Here's the drawing with two shaded views (mm, measured from the low corner). I have some questions. A direction names the side the tool comes from. Coordinates: 2 decimals unless noted, no trailing zeros. Write each loop counter-clockwise with the first axis right and the second up, starting at its lowest first coordinate (ties: lowest second). Pieces come first, ordered by that corner, then holes. Notation, with made-up numbers: (80, 19.5) -> (93, 19.5) arc R23 cw to (93, 36.5) -> close; hole circle Ø1 at (1, 51.25). An arc over 180 degrees is marked (long way). Use one line per item in the form item = value.
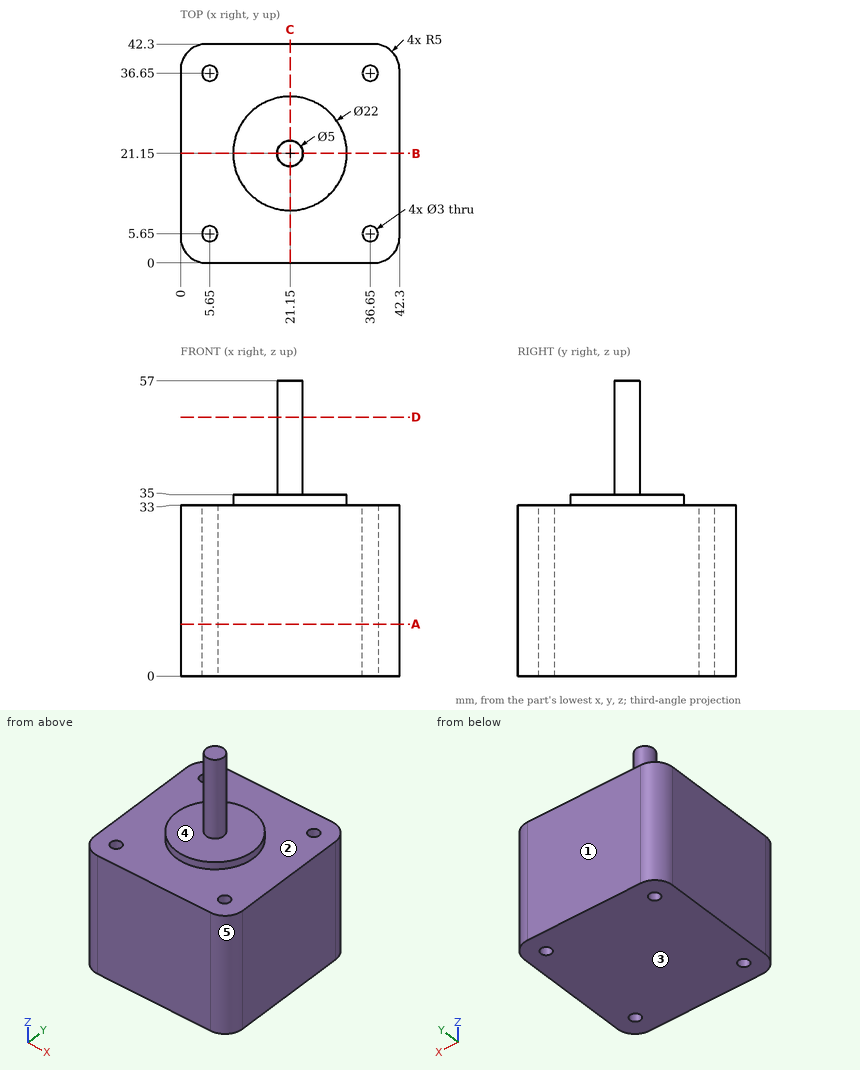
Q1. Thinking about a two-plate mould opening in Z: for the marked faces 3, 4 and 5, which applies, released by +Z, released by -Z, zero draft, split by the parting line, or undercut?
Return value:
face_3 = released by -Z
face_4 = released by +Z
face_5 = zero draft
Q2. For the marked faces 1 and 2, which set-ups out of +Z, -Z, +X, -X, +Y, -Y let a thin tool reach every point of the face, with its end or its side?
Return value:
face_1 = +Z, -Z, +X, -X, +Y
face_2 = +Z
Q3. Suppose I cut it at B-B (y = 21.15). Write out the boundary of the cut face in (x, z), then the cut area to 3 significant figures.
Return value:
outline = (0, 0) -> (42.3, 0) -> (42.3, 33) -> (32.15, 33) -> (32.15, 35) -> (23.65, 35) -> (23.65, 57) -> (18.65, 57) -> (18.65, 35) -> (10.15, 35) -> (10.15, 33) -> (0, 33) -> close
area = 1,550 mm2
Q4. Suppose I cut it at D-D (z = 50). Write out the boundary of the cut face in (x, y).
Return value:
outline = circle Ø5 at (21.15, 21.15)
Q5. Will these pins go through, and if not, where does the flat tip stop? pin 1 (10 mm diameter, centred on x = 18, z = 41.5, fed in from -Y); pin 2 (12 mm diameter, centred on x = 10, z = 50, fed in from +Y); pin 3 (4 mm diameter, centred on x = 5.65, y = 36.65, fed in from +Z).
Return value:
pin_1 = 18.65
pin_2 = through
pin_3 = 33
Q6. If I drill on line 1 (Y direction, x = 5.65, z = 18); line 2 (Y direction, x = 36, z = 9); line 3 (Z direction, x = 35, y = 32), over which ranges is the centre line in solid material (lowest first)? Write a range as from..to.
Return value:
line_1 = 0..4.15, 7.15..35.15, 38.15..42.3
line_2 = 0..4.3, 7..35.3, 38..42.3
line_3 = 0..33
Q7. Suppose I cut it at A-A (z = 10). Write out the boundary of the cut face in (x, y), then the cut area to 3 significant figures.
Return value:
outline = (0, 5) arc R5 ccw to (5, 0) -> (37.3, 0) arc R5 ccw to (42.3, 5) -> (42.3, 37.3) arc R5 ccw to (37.3, 42.3) -> (5, 42.3) arc R5 ccw to (0, 37.3) -> close; hole circle Ø3 at (5.65, 5.65); hole circle Ø3 at (5.65, 36.65); hole circle Ø3 at (36.65, 5.65); hole circle Ø3 at (36.65, 36.65)
area = 1,740 mm2
